Read the model definition and answer for the solid it produces. Units are mm, in the model's axes. Face numbers are marked on the shaded views. A direction names the side the tool comes from. Coordinates: 2 decimals unless noted, no trailing zeros. Order: outer loops, then holes, each group sorted by start corner. A loop starts at its lowest first (then second) coordinate and runs counter-clockwise, first axis right, second up. Notation, with made-up numbers: (61.5, 39.25) - (82.5, 39.25) arc R28 cw to (82.5, 73.25) - close; hole circle Ø10 at (-3, 73). An arc over 180 degrees is marked (long way). Use one line per item in the form item = value. Start each with the question number.
from build123d import *

# Parameters (mm, degrees)
SKETCH2_W               = 27
SKETCH2_H               = 32
SKETCH2_R               = 9
BOSS_EXTRUDE1_DEPTH     = 6
SKETCH3_W               = 27
SKETCH3_H               = 32
SKETCH3_W_2             = 25
SKETCH3_H_2             = 30
BOSS_EXTRUDE2_DEPTH     = 3
SKETCH1_R               = 1.5
CUT_EXTRUDE1_DEPTH      = 7
CUT_EXTRUDE1_DEPTH_BACK = 4
BOSS_EXTRUDE4_DEPTH     = 9
MIRROR2_COPY_1_DEPTH    = 9
SKETCH6_R               = 2.8
CUT_EXTRUDE2_DEPTH      = 2
MIRROR4_COPY_1_SKETCH_R = 2.8
MIRROR4_COPY_1_DEPTH    = 2
FILLET1_R               = 1
SKETCH11_W              = 9.5
SKETCH11_H              = 9.5
CUT_EXTRUDE3_DEPTH      = 2
MIRROR6_COPY_1_SKETCH_W = 9.5
MIRROR6_COPY_1_SKETCH_H = 9.5
MIRROR6_COPY_1_DEPTH    = 2
FILLET2_R               = 1


with BuildPart() as part:
    # Sketch2 → Boss-Extrude1 (new body)
    with BuildSketch(Plane(origin=(0, 0, 0), x_dir=(1, 0, 0), z_dir=(0, 1, 0))):
        Rectangle(SKETCH2_W, SKETCH2_H)
        Circle(SKETCH2_R, mode=Mode.SUBTRACT)
    extrude(amount=BOSS_EXTRUDE1_DEPTH)

    # Sketch3 → Boss-Extrude2 (add)
    with BuildSketch(Plane.XZ):
        Rectangle(SKETCH3_W, SKETCH3_H)
        Rectangle(SKETCH3_W_2, SKETCH3_H_2, mode=Mode.SUBTRACT)
    extrude(amount=BOSS_EXTRUDE2_DEPTH)

    # Sketch1 → Cut-Extrude1 (cut, two sides)
    with BuildSketch(Plane(origin=(0, 0, 0), x_dir=(1, 0, 0), z_dir=(0, 1, 0))) as cut_extrude1_sk:
        with Locations((-12.5, 12)):
            Circle(SKETCH1_R)
        with Locations((12.5, 12)):
            Circle(SKETCH1_R)
        with Locations((-12.5, -12)):
            Circle(SKETCH1_R)
        with Locations((12.5, -12)):
            Circle(SKETCH1_R)
    extrude(amount=CUT_EXTRUDE1_DEPTH, mode=Mode.SUBTRACT)
    extrude(cut_extrude1_sk.sketch, amount=-CUT_EXTRUDE1_DEPTH_BACK, mode=Mode.SUBTRACT)

    # Sketch5 → Boss-Extrude4 (add)
    with BuildSketch(Plane.XZ.offset(3)):
        with BuildLine():
            Line((13.5, -10.881966011), (13.5, -9.708712153))
            ThreePointArc((13.5, -9.708712153), (10, -12), (13.5, -14.291287847))
            Line((13.5, -14.291287847), (13.5, -13.118033989))
            ThreePointArc((13.5, -13.118033989), (11, -12), (13.5, -10.881966011))
        make_face()
    boss_extrude4 = extrude(amount=-BOSS_EXTRUDE4_DEPTH)

    # Mirror1: Boss-Extrude4 across plane
    add(boss_extrude4.mirror(Plane(origin=(0, 0, 0), x_dir=(0, 0, 1), z_dir=(1, 0, 0))))

    # Mirror2: Boss-Extrude4 across plane
    add(boss_extrude4.mirror(Plane.XY))

    # Mirror2 copy 1 sketch → Mirror2 copy 1 (add)
    with BuildSketch(Plane(origin=(0, -3, 0), x_dir=(-1, 0, 0), z_dir=(0, -1, 0))):
        with BuildLine():
            Line((13.5, -10.881966011), (13.5, -9.708712153))
            ThreePointArc((13.5, -9.708712153), (10, -12), (13.5, -14.291287847))
            Line((13.5, -14.291287847), (13.5, -13.118033989))
            ThreePointArc((13.5, -13.118033989), (11, -12), (13.5, -10.881966011))
        make_face()
    extrude(amount=-MIRROR2_COPY_1_DEPTH)

    # Sketch6 → Cut-Extrude2 (cut)
    with BuildSketch(Plane(origin=(0, 6, 0), x_dir=(1, 0, 0), z_dir=(0, 1, 0))):
        with Locations((12.5, 12)):
            Circle(SKETCH6_R)
    cut_extrude2 = extrude(amount=-CUT_EXTRUDE2_DEPTH, mode=Mode.SUBTRACT)

    # Mirror3: Cut-Extrude2 across plane
    add(cut_extrude2.mirror(Plane(origin=(0, 0, 0), x_dir=(0, 0, 1), z_dir=(1, 0, 0))), mode=Mode.SUBTRACT)

    # Mirror4: Cut-Extrude2 across plane
    add(cut_extrude2.mirror(Plane.XY), mode=Mode.SUBTRACT)

    # Mirror4 copy 1 sketch → Mirror4 copy 1 (cut)
    with BuildSketch(Plane(origin=(0, 6, 0), x_dir=(-1, 0, 0), z_dir=(0, 1, 0))):
        with Locations((12.5, 12)):
            Circle(MIRROR4_COPY_1_SKETCH_R)
    extrude(amount=-MIRROR4_COPY_1_DEPTH, mode=Mode.SUBTRACT)

    # Fillet1
    fillet1_edges = [part.edges().sort_by_distance(p)[0] for p in [
        (-13.5, 6, -15.307669683),
        (13.5, 6, -15.307669683),
        (0, 6, 16),
        (-13.5, 6, 0),
        (13.5, 6, 0),
        (-13.5, 6, 15.307669683),
        (13.5, 6, 15.307669683),
        (0, 6, -16),
    ]]
    fillet(fillet1_edges, radius=FILLET1_R)

    # Sketch11 → Cut-Extrude3 (cut)
    with BuildSketch(Plane(origin=(0, 6, 0), x_dir=(1, 0, 0), z_dir=(0, 1, 0))):
        with Locations((-12.5, -12)):
            Rectangle(SKETCH11_W, SKETCH11_H)
    cut_extrude3 = extrude(amount=-CUT_EXTRUDE3_DEPTH, mode=Mode.SUBTRACT)

    # Mirror5: Cut-Extrude3 across plane
    add(cut_extrude3.mirror(Plane(origin=(0, 0, 0), x_dir=(0, 0, 1), z_dir=(1, 0, 0))), mode=Mode.SUBTRACT)

    # Mirror6: Cut-Extrude3 across plane
    add(cut_extrude3.mirror(Plane.XY), mode=Mode.SUBTRACT)

    # Mirror6 copy 1 sketch → Mirror6 copy 1 (cut)
    with BuildSketch(Plane(origin=(0, 6, 0), x_dir=(-1, 0, 0), z_dir=(0, 1, 0))):
        with Locations((-12.5, -12)):
            Rectangle(MIRROR6_COPY_1_SKETCH_W, MIRROR6_COPY_1_SKETCH_H)
    extrude(amount=-MIRROR6_COPY_1_DEPTH, mode=Mode.SUBTRACT)

    # Fillet2
    fillet2_edges = [part.edges().sort_by_distance(p)[0] for p in [
        (-7.75, 4.5, 16),
        (-13.5, 4.5, 7.25),
        (-7.75, 6, 11.125),
        (-10.125, 6, 7.25),
        (7.75, 6, 11.125),
        (10.125, 6, 7.25),
        (7.75, 4.5, 16),
        (13.5, 4.5, 7.25),
        (13.5, 4.5, -7.25),
        (7.75, 4.5, -16),
        (7.75, 6, -11.125),
        (10.125, 6, -7.25),
        (-7.75, 6, -11.125),
        (-10.125, 6, -7.25),
        (-7.75, 4.5, -16),
        (-13.5, 4.5, -7.25),
    ]]
    fillet(fillet2_edges, radius=FILLET2_R)


solid = part.part
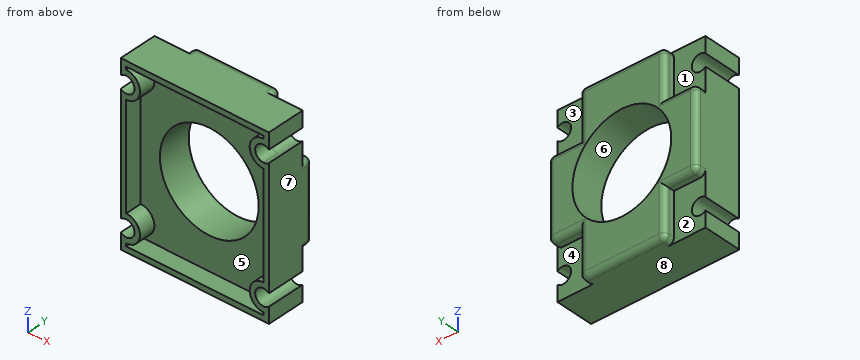
Q1. Which of the six approach directions +Z, -Z, +X, -X, +Y, -Y give full straight-line access (tool end or side, diameter ignored) to the marked faces 1, 2, 3, 4 and 5?
Q2. A cutting plane is placed at B-B (x = 0). Give the vertices of the cut face in (y, z), then the cut area to 3 significant figures.
Q3. Given P1, Ø2, axis at x = 10, z = -12.5, coming from the +Y side; P2, Ø2.5, axis at x = 12.5, z = -12, coming from the -Y side; P3, Ø1.5, axis at x = 10, z = -8, coming from the -Y side, each flat-ended and moving along its own axis, determine where each tip first touches the part or whether it passes through.
Q4. A cutting plane is placed at D-D (z = 12). Give the vertices of the cut face in (x, y), then the cut area to 3 significant figures.
Q5. A cutting plane is placed at C-C (z = 0). Give the vertices of the cut face in (x, y), then the cut area to 3 significant figures.
Q6. A cutting plane is placed at A-A (y = 3). Give the vertices of the cut face in (x, z), then the cut area to 3 significant figures.
Q7. Consider probe 1 along Z at (x, y) = (-12.5, 2.25); probe 2 along Z at (x, y) = (-7.75, -1.5); probe 3 along X at (y, z) = (-1, -12). Determine where each line is inside the solid, lowest interval first.
Q8. For a pull along Z with two mould halves and no side action, classify the marked faces 6, 7 and 8 as +Z half, -Z half, draft (parallel to the pull), parting line (faces both ways), or undercut.
Result sheet:
q1.face_1 = +Z, -X, +Y
q1.face_2 = -Z, -X, +Y
q1.face_3 = +Z, +X, +Y
q1.face_4 = -Z, +X, +Y
q1.face_5 = -Y
q2.outline = (-3, -16) - (5, -16) arc R1 ccw to (6, -15) - (6, -9) - (0, -9) - (0, -15) - (-3, -15) - close; (-3, 15) - (0, 15) - (0, 9) - (6, 9) - (6, 15) arc R1 ccw to (5, 16) - (-3, 16) - close
q2.area = 89.6 mm^2
q3.P1 = 4
q3.P2 = through
q3.P3 = 0
q4.outline = (-11, -3) - (-10, -3) - (-10, 0) - (10, 0) - (10, -3) - (11, -3) - (11, 4) - (7.75, 4) - (7.75, 5) arc R1 ccw to (6.75, 6) - (-6.75, 6) arc R1 ccw to (-7.75, 5) - (-7.75, 4) - (-11, 4) - close
q4.area = 125 mm^2
q5.outline = (-13.5, -3) - (-12.5, -3) - (-12.5, 0) - (-9, 0) - (-9, 6) - (-12.5, 6) arc R1 ccw to (-13.5, 5) - close; (9, 0) - (12.5, 0) - (12.5, -3) - (13.5, -3) - (13.5, 5) arc R1 ccw to (12.5, 6) - (9, 6) - close
q5.area = 59.6 mm^2
q6.outline = (-13.5, -16) - (13.5, -16) - (13.5, -13.12) arc R1.5 cw (long way) to (13.5, -10.88) - (13.5, 10.88) arc R1.5 cw (long way) to (13.5, 13.12) - (13.5, 16) - (-13.5, 16) - (-13.5, 13.12) arc R1.5 cw (long way) to (-13.5, 10.88) - (-13.5, -10.88) arc R1.5 cw (long way) to (-13.5, -13.12) - close; hole circle Ø18 at (0, 0)
q6.area = 584 mm^2
q7.probe_1 = -16 to -13.5, -10.5 to 10.5, 13.5 to 16
q7.probe_2 = -16 to -15, 15 to 16
q7.probe_3 = -11 to -10, 10 to 11
q8.face_6 = undercut
q8.face_7 = draft
q8.face_8 = -Z half
